Could you check a few things on this drawing? It's one solid part, dimensions in mm from its lowest x, y, z. A direction names the side the tool comes from. Give positions to 0.01 mm unless a question says otherwise; leave off trailing zeros. Order: outer loops, then holes, each group sorted by start corner. A loop starts at its lowest first (then second) coordinate and runs counter-clockwise, first axis right, second up. Notation, with made-up numbers: (25, 13) -> (84, 13) arc R19 ccw to (84, 48) -> close; hole circle Ø10 at (38.5, -12). An arc over 180 degrees is marked (long way). Answer as CSV lines item,"result".
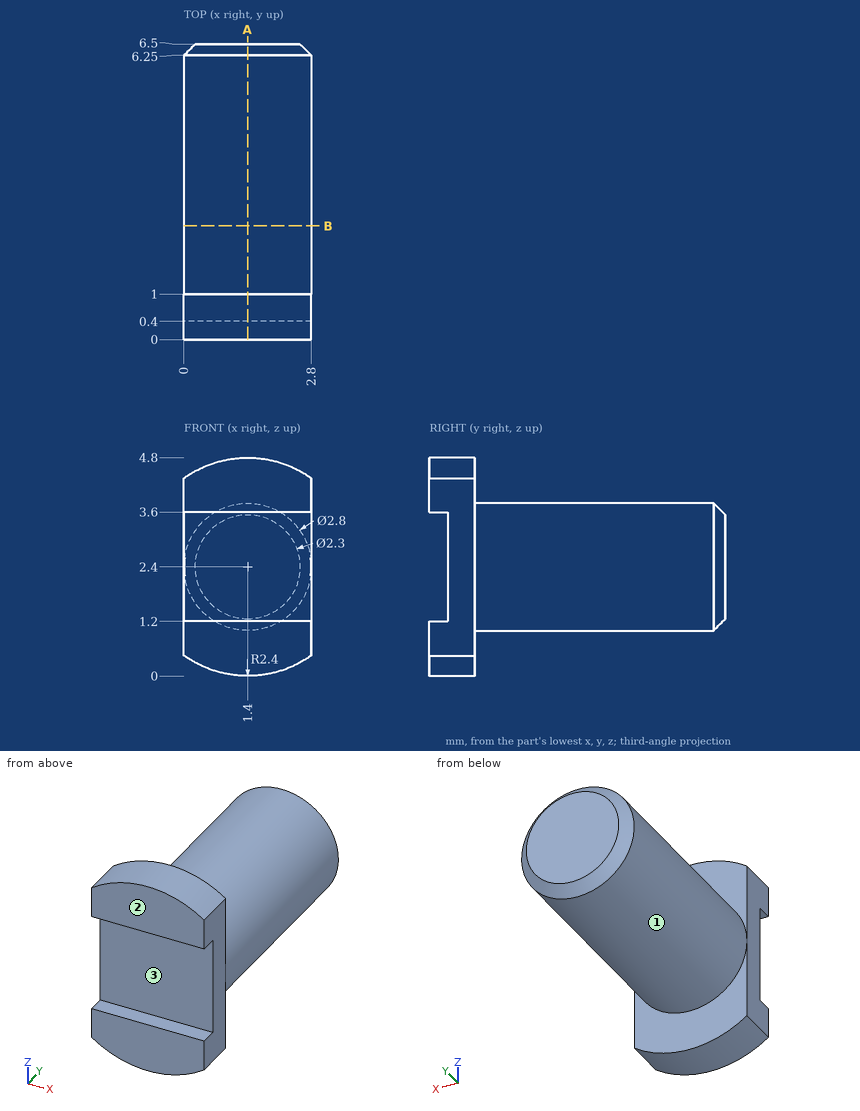
Item 1: Please list where these lines run through material, in increasing order: line 1 along Y through (x, z) = (0.75, 0.8); line 2 along Z through (x, y) = (0.6, 1.25); line 3 along Y through (x, z) = (2.4, 2.35).
Numbers:
line 1,"y = 0 to 1"
line 2,"z = 1.25 to 3.55"
line 3,"y = 0.4 to 6.5"
Item 2: For the marked faces 1, 2 and 3, which set-ups out of +Z, -Z, +X, -X, +Y, -Y let a thin tool reach every point of the face, with its end or its side?
Numbers:
face 1,"+Y"
face 2,"+Z, -Z, +X, -X, -Y"
face 3,"+X, -X, -Y"
Item 3: Imagine slicing it at A-A, the plane x = 1.4. Please give me the cut outline in (y, z).
Numbers:
outline,"(0, 0) -> (1, 0) -> (1, 1) -> (6.25, 1) -> (6.5, 1.25) -> (6.5, 3.55) -> (6.25, 3.8) -> (1, 3.8) -> (1, 4.8) -> (0, 4.8) -> (0, 3.6) -> (0.4, 3.6) -> (0.4, 1.2) -> (0, 1.2) -> close"
Item 4: For pin 1 (1 mm diameter, centred on x = 1.5, y = 2, fed in from -Z); pin 2 (1 mm diameter, centred on x = 1.5, z = 4, fed in from -Y); pin 3 (0.7 mm diameter, centred on x = 1.5, z = 4, fed in from +Y), each with a flat end and sliding along its axis, tell me the tip position at first contact or that it passes through.
Numbers:
pin 1,"stops at z = 1"
pin 2,"stops at y = 0"
pin 3,"stops at y = 6.4"
Item 5: Imagine slicing it at B-B, the plane y = 2.5. Please give me the cut outline in (x, z).
Numbers:
outline,"circle Ø2.8 at (1.4, 2.4)"
